from build123d import *
from OCP.BRepFilletAPI import BRepFilletAPI_MakeChamfer

# Parameters (mm, degrees)
SKETCH_1_W       = 80
SKETCH_1_H       = 80
EXTRUDE_1_DEPTH  = 20
SKETCH_2_R       = 30
EXTRUDE_2_DEPTH  = 5
CHAMFER_1_SIZE   = 20
CHAMFER_1_SIZE_2 = 5


with BuildPart() as part:
    # Эскиз1 → Бобышка-Вытянуть1 (new body)
    with BuildSketch(Plane(origin=(0, 0, 0), x_dir=(1, 0, 0), z_dir=(0, 1, 0))):
        Rectangle(SKETCH_1_W, SKETCH_1_H)
    extrude(amount=EXTRUDE_1_DEPTH)

    # Эскиз2 → Бобышка-Вытянуть2 (add)
    with BuildSketch(Plane(origin=(0, 20, 0), x_dir=(1, 0, 0), z_dir=(0, 1, 0))):
        with Locations(Location((0, 0, 0), (0, 0, 270))):
            Circle(SKETCH_2_R)
    extrude(amount=EXTRUDE_2_DEPTH)

    # Фаска1
    chamfer_1_edges_1 = [part.edges().sort_by_distance(p)[0] for p in [
        (40, 20, 0),
    ]]
    chamfer_1_side_1 = [part.faces().sort_by_distance(p)[0] for p in [
        (40, 19.9, 0),
    ]]
    chamfer_1_edges_2 = [part.edges().sort_by_distance(p)[0] for p in [
        (0, 20, -40),
    ]]
    chamfer_1_side_2 = [part.faces().sort_by_distance(p)[0] for p in [
        (0, 20, -39.9),
    ]]
    chamfer_1_edges_3 = [part.edges().sort_by_distance(p)[0] for p in [
        (-40, 20, 0),
    ]]
    chamfer_1_side_3 = [part.faces().sort_by_distance(p)[0] for p in [
        (-40, 19.9, 0),
    ]]
    chamfer_1_edges_4 = [part.edges().sort_by_distance(p)[0] for p in [
        (0, 20, 40),
    ]]
    chamfer_1_side_4 = [part.faces().sort_by_distance(p)[0] for p in [
        (0, 19.9, 40),
    ]]
    chamfer_1 = BRepFilletAPI_MakeChamfer(part.part.solid().wrapped)
    for e in chamfer_1_edges_1:
        chamfer_1.Add(CHAMFER_1_SIZE - 0.0001, CHAMFER_1_SIZE_2 - 0.0001, e.wrapped, chamfer_1_side_1[0].wrapped)
    for e in chamfer_1_edges_2:
        chamfer_1.Add(CHAMFER_1_SIZE_2 - 0.0001, CHAMFER_1_SIZE - 0.0001, e.wrapped, chamfer_1_side_2[0].wrapped)
    for e in chamfer_1_edges_3:
        chamfer_1.Add(CHAMFER_1_SIZE - 0.0001, CHAMFER_1_SIZE_2 - 0.0001, e.wrapped, chamfer_1_side_3[0].wrapped)
    for e in chamfer_1_edges_4:
        chamfer_1.Add(CHAMFER_1_SIZE - 0.0001, CHAMFER_1_SIZE_2 - 0.0001, e.wrapped, chamfer_1_side_4[0].wrapped)
    add(Compound.cast(chamfer_1.Shape()), mode=Mode.REPLACE)  # a hair under: the kernel refuses the full size


solid = part.part
Read the model definition and answer for the solid it produces. Units are mm, in the model's axes. Coordinates: 2 decimals unless noted, no trailing zeros. Loops run counter-clockwise (first coordinate to the right, second up) from the corner with the lowest first, then second, coordinate; pieces in that order, holes last. Notation, with made-up numbers: (-10, -27.75) - (0, -27.75) arc R24 cw to (0, -14.75) - close; hole circle Ø7 at (24.25, 9). An arc over 180 degrees is marked (long way). Answer in a Markdown table with one row per item.
Q1. Given P1, Ø8, axis at x = 18, y = 15, coming from the -Z side; P2, Ø3, axis at y = 3.5, z = 23.5, coming from the +X side; P3, Ø2, axis at y = 17.5, z = -22, coming from the +X side, each flat-ended and moving along its own axis, determine where each tip first touches the part or whether it passes through.
Here are the results:
| item | result |
|---|---|
| P1 | stops at z = -37.25 |
| P2 | stops at x = 39.5 |
| P3 | stops at x = 35.88 |
Q2. Straight lines are drawn through the part: line 1 along Y through (x, z) = (32, -3); line 2 along Z through (x, y) = (-17.5, 21); line 3 along Z through (x, y) = (-20, 11.5). For each, find the intervals that lie inside material, in ascending order. Write a range as [from, to].
Here are the results:
| item | result |
|---|---|
| line 1 | y = [0, 20] |
| line 2 | z = [-24.37, 24.37] |
| line 3 | z = [-37.13, 37.13] |
Q3. The mould has two halves that part along X. Classify faces 1 (the cylindrical face through (1.32, 22.46, -29.97)), 2 (the flat face through (-37.465, 10.14, 0.56)), 3 (the flat face through (31, 20, 0)): pulls with the +X half, pulls with the -X half, needs draft (parallel to the pull), parting line crosses it, or undercut.
Here are the results:
| item | result |
|---|---|
| face 1 | parting line crosses it |
| face 2 | pulls with the -X half |
| face 3 | needs draft |
Q4. Find section C-C on y = 21.5. Write down the section's boundary in (x, z), plus the area to 3 significant figures.
Here are the results:
| item | result |
|---|---|
| outline | circle Ø60 at (0, 0) |
| area | 2,830 mm^2 |
